Work out the finished part from the listing and answer in its coordinate system (mm). A direction names the side the tool comes from. Give positions to 0.01 mm unless a question says otherwise; leave off trailing zeros. Order: outer loops, then holes, each group sorted by start corner. A loop starts at its lowest first (then second) coordinate and runs counter-clockwise, first axis right, second up.
Autodesk Inventor part; units mm, degrees
ref_plane "YZ Plane" through (0, 0, 0) normal (1, 0, 0) x (0, 1, 0)
ref_plane "XZ Plane" through (0, 0, 0) normal (0, 1, 0) x (-1, 0, 0)
ref_plane "XY Plane" through (0, 0, 0) normal (0, 0, 1) x (1, 0, 0)
sketch "Sketch1" plane through (0, 0, 0) normal (0, 0, 1) x (1, 0, 0)
  circle A0 centre (-10, 0) radius 1.5
  circle A1 centre (10, 0) radius 1.5
  circle A2 centre (-10, -20) radius 1.5
  circle A3 centre (10, -20) radius 1.5
  line L0 (-15, 10) -> (15, 10)
  line L1 (15, 10) -> (15, -30)
  line L2 (15, -30) -> (-15, -30)
  line L3 (-15, -30) -> (-15, 10)
  point P0 (0, 0)
  dimension "d0" = 3
  dimension "d1" = 3
  dimension "d2" = 20
  dimension "d3" = 10
  dimension "d4" = 3
  dimension "d5" = 3
  dimension "d6" = 20
  dimension "d7" = 20
  dimension "d8" = 20
  dimension "d9" = 10
  dimension "d10" = 30
  dimension "d11" = 15
  dimension "d12" = 40
  dimension "d13" = 10
extrude "Extrusion1" add sketch "Sketch1" along normal blind 4
sketch "Sketch2" plane through (0, 0, 4) normal (0, 0, 1) x (1, 0, 0)
  line L0 (0, 15.4421) -> (0, -37.5419) construction
  line L1 (-4, 15.4421) -> (-4, -37.5419) construction
  line L2 (-15, -30) -> (15, -30) construction
  line L3 (15, 10) -> (-15, 10)
  line L4 (9, -30) -> (9, 10)
  line L5 (7, 10) -> (7, -30)
  line L6 (7, 10) -> (9, 10)
  line L7 (7, -30) -> (9, -30)
  line L8 (6.3, 15.4421) -> (6.3, 10) construction
  line L9 (6.3, -30) -> (6.3, -37.5419) construction
  line L10 (-15, 10) -> (-15, -30)
  point P0 (0, 0)
  dimension "d16" = 4
  dimension "d96" = 0
  dimension "d97" = 0
  dimension "d141" = 22
extrude "Extrusion2" add sketch "Sketch2" along normal blind 6
sketch "Sketch4" plane through (0, 0, 10) normal (0, 0, 1) x (1, 0, 0)
  circle A0 centre (10, 0) radius 2.75
  circle A1 centre (10, -20) radius 1.5
  circle A2 centre (10, -20) radius 2.75
  point P0 (0, 0)
  point P1 (8.5, 0)
  point P2 (8.5, -20)
  dimension "d37" = 5.5
  dimension "d38" = 5.5
extrude "Extrusion3" cut sketch "Sketch4" against normal up to surface (6 mm away) contours A0 | A1 | A2
sketch "Sketch5" plane through (0, 0, 4) normal (0, 0, 1) x (1, 0, 0)
  line L0 (-4, 15.4421) -> (-4, -37.5419) construction
  line L1 (15, -30) -> (-15, -30)
  line L2 (15, 10) -> (-15, 10)
  line L3 (-3.3, 10) -> (5, 10)
  line L4 (5, -30) -> (-3.3, -30)
  line L5 (-3.3, -30) -> (-3.3, 10)
  line L6 (-2, 7) -> (5, 7)
  line L7 (5, -27) -> (-2, -27)
  line L8 (-2, -27) -> (-2, 7)
  line L9 (5, 10) -> (5, 7)
  line L10 (5, -27) -> (5, -30)
  line L11 (7, 10) -> (7, -30)
  point P0 (0, 0)
  point P1 (6.3, 10)
  point P2 (6.3, -30)
  dimension "d111" = 0.7
  dimension "d112" = 3
  dimension "d115" = 3
  dimension "d116" = 1.3
  dimension "d117" = 2
  dimension "d118" = 2
  dimension "d139" = 0
  dimension "d140" = 0
extrude "Extrusion4" add sketch "Sketch5" along normal up to surface (6 mm away) contours L1 L5 L2 L9 L6 L8 L7 L10
sketch "Sketch8" plane through (0, 0, 0) normal (0, 0, -1) x (-1, 0, 0)
  line L0 (27, -15) -> (-27, -15)
  line L1 (-27, -15) -> (-27, -5)
  line L2 (-27, -5) -> (27, -5)
  line L3 (27, -5) -> (27, -15)
  line L4 (15, 10) -> (-15, 10)
  line L5 (-15, -30) -> (15, -30)
  circle A0 centre (23, -10) radius 1.5
  circle A1 centre (-23, -10) radius 1.5
  point P0 (0, 0)
  dimension "d77" = 10
  dimension "d78" = 40
  dimension "d79" = 15
  dimension "d80" = 3
  dimension "d81" = 3
  dimension "d82" = 46
  dimension "d83" = 54
  dimension "d84" = 23
  dimension "d85" = 27
extrude "Extrusion5" add sketch "Sketch8" against normal up to surface (4 mm away)
sketch "Sketch3" plane through (0, 0, 4) normal (0, 0, 1) x (1, 0, 0)
  circle A0 centre (2, -2) radius 1.25
  circle A1 centre (2, -15) radius 1.25
  line L0 (-15, -30) -> (15, -30)
  line L1 (15, 10) -> (-15, 10)
  point P0 (0, 0)
  point P1 (7, -30)
  point P2 (6.3, 10)
  dimension "d23" = 2.5
  dimension "d24" = 2.5
  dimension "d25" = 15
  dimension "d26" = 2
  dimension "d27" = 2
  dimension "d28" = 12
hole "Hole1" at (2, -2, 4) at (2, -15, 4) direction (0, 0, -1) diameter 2.5 end through all
fillet "Fillet5" [suppressed]
fillet "Fillet7" [suppressed]
sketch "Sketch11" plane through (0, 0, 0) normal (0, 0, -1) x (-1, 0, 0)
  line L0 (15, -15) -> (13.5, -15)
  line L1 (13.5, -5) -> (15, -5)
  line L2 (-15, -5) -> (-13.5, -5)
  line L3 (-13.5, -15) -> (-15, -15)
  line L4 (15, -30) -> (15, -15)
  line L5 (-15, -15) -> (-15, -30)
  line L6 (-15, 10) -> (-15, -5)
  line L7 (15, -5) -> (15, 10)
  line L8 (-15, -30) -> (-13.5, -30)
  line L9 (13.5, -30) -> (15, -30)
  line L10 (-13.5, -30) -> (-13.5, -15)
  line L11 (-13.5, -5) -> (-13.5, 10)
  line L12 (13.5, 10) -> (13.5, -5)
  line L13 (13.5, -15) -> (13.5, -30)
  line L14 (15, 10) -> (13.5, 10)
  line L15 (-15, 10) -> (15, 10)
  line L16 (-15, 10) -> (-13.5, 10)
  point P0 (0, 0)
  dimension "d121" = 27
extrude "Extrusion7" cut sketch "Sketch11" against normal through all
fillet "Fillet9" radius 3 12 edges at (-27, -15, 2) (-13.5, -30, 2) (13.5, -30, 2) (-27, -5, 2) (-13.5, -5, 2) (-13.5, 10, 2) (13.5, -15, 2) (27, -15, 2) (27, -5, 2) (13.5, -5, 2) (13.5, 10, 2) (-13.5, -15, 2)
sketch "Sketch12" plane through (4, -30, 4) normal (0, -1, 0) x (1, 0, 0)
  line L0 (1, 6) -> (-7.3, 6)
  circle A0 centre (-2, 3) radius 1.5
  line L1 (5, 0) -> (6.5, 0)
  line L2 (6.5, -4) -> (-14.5, -4)
  line L3 (6.5, 0) -> (6.5, -4)
  line L4 (-14.5, -4) -> (-14.5, 0)
  line L5 (-7.3, 0) -> (-7.3, 6)
  line L6 (-14.5, 0) -> (-7.3, 0)
  line L7 (5, 0) -> (5, 6)
  line L8 (3, 6) -> (5, 6)
  line L9 (3, 0) -> (3, 6)
  line L10 (1, 0) -> (3, 0)
  line L11 (1, 0) -> (1, 6)
  point P0 (-4, -4)
  dimension "d126" = 3
  dimension "d129" = 3
extrude "Extrusion8" [suppressed]
sketch "Sketch14" plane through (0, 0, 0) normal (0, 0, -1) x (-1, 0, 0)
  line L0 (10.5, 10) -> (-10.5, 10)
  line L1 (-1.2, 10) -> (1.2, 10)
  line L2 (1.2, 10) -> (1.2, 24)
  line L3 (1.2, 24) -> (-1.2, 24)
  line L4 (-1.2, 24) -> (-1.2, 10)
  point P0 (0, 0)
  dimension "d142" = 14
  dimension "d143" = 1.2
  dimension "d144" = 1.2
extrude "Extrusion10" add sketch "Sketch14" against normal blind 10
fillet "Fillet10" radius 3 2 edges at (-1.2, 10, 5) (1.2, 10, 5)
fillet "Fillet11" radius 1 2 edges at (-1.2, 24, 5) (1.2, 24, 5)
sketch "Sketch13" plane through (-10.5, -30, 0) normal (0, -1, 0) x (1, 0, 0)
  line L0 (21, 4) -> (21, 0)
  line L1 (0, 4) -> (21, 4)
  line L2 (0, 0) -> (0, 4)
  line L3 (21, 0) -> (0, 0)
  circle A0 centre (10.5, 2) radius 1.5
  point P0 (10.5, 0)
  dimension "d132" = 3
  dimension "d133" = 21
  dimension "d134" = 4
  dimension "d135" = 2
  dimension "d136" = 10.5
sketch "Sketch9" plane through (0, 0, 4) normal (0, 0, 1) x (1, 0, 0)
  circle A0 centre (-10, 0) radius 1.5
  circle A1 centre (2, -2) radius 1.25
  circle A2 centre (10, 0) radius 1.5
  circle A3 centre (23, -10) radius 1.5
  circle A4 centre (10, -20) radius 1.5
  circle A5 centre (2, -15) radius 1.25
  circle A6 centre (-10, -20) radius 1.5
  circle A7 centre (-23, -10) radius 1.5
  point P0 (0, 0)
equation "\"d7\" = d6"
equation "\"d8\" = d2"
equation "\"d37\" = d38"
equation "\"d115\" = d112"
equation "\"d79\" = -0.5 * d77 + 0.5 * d78"
properties part number "vertical carriage"
1. The part is cut by section D-D (y = 5). Write down the section's boundary in (x, z).
Findings below:
outline: (-13.5, 0) - (13.5, 0) - (13.5, 4) - (9, 4) - (9, 10) - (7, 10) - (7, 4) - (-2, 4) - (-2, 10) - (-3.3, 10) - (-3.3, 4) - (-13.5, 4) - close
2. The part is cut by section A-A (z = 5.75). Write down the section's boundary in (x, y).
Findings below:
outline: (-3.3, -30) - (5, -30) - (5, -27) - (-2, -27) - (-2, 7) - (5, 7) - (5, 10) - (4.2, 10) arc R3 cw to (1.2, 13) - (1.2, 23) arc R1 ccw to (0.2, 24) - (-0.2, 24) arc R1 ccw to (-1.2, 23) - (-1.2, 13) arc R3 cw to (-3.3, 10.14) - close; (7, -30) - (9, -30) - (9, -22.56) arc R2.75 cw to (9, -17.44) - (9, -2.56) arc R2.75 cw to (9, 2.56) - (9, 10) - (7, 10) - close
3. The part is cut by section B-B (y = -20). Write down the section's boundary in (x, z).
Findings below:
outline: (-13.5, 0) - (-11.5, 0) - (-11.5, 4) - (-13.5, 4) - close; (-8.5, 0) - (8.5, 0) - (8.5, 4) - (7.25, 4) - (7.25, 10) - (7, 10) - (7, 4) - (-2, 4) - (-2, 10) - (-3.3, 10) - (-3.3, 4) - (-8.5, 4) - close; (11.5, 0) - (13.5, 0) - (13.5, 4) - (11.5, 4) - close
4. Straight lines are drawn through the part: probe 1 along Y at (x, z) = (10, 1.05); probe 2 along Y at (x, z) = (-23, 1.5); probe 3 along X at (y, z) = (-9, 4.25). For each, find the intervals that lie inside material, in ascending order.
Findings below:
probe 1: y = -30 to -21.5, -18.5 to -1.5, 1.5 to 10
probe 2: y = -15 to -11.5, -8.5 to -5
probe 3: x = -3.3 to -2, 7 to 9
5. Which of the six approach directions +Z, -Z, +X, -X, +Y, -Y give full straight-line access (tool end or side, diameter ignored) to faces 1 (the face through (-13.5, 3, 2)), 2 (the face through (20, -15, 2)), 3 (the face through (1, 7, 7)), 4 (the face through (13.5, 2, 2))?
Findings below:
face 1: +Z, -Z, -X, +Y
face 2: +Z, -Z, +X, -Y
face 3: +Z
face 4: +Z, -Z, +X, +Y
6. The mould has two halves that part along X. Classify faces 5 (the face through (9, -10, 7)), 6 (the face through (2, -10, 4)), 7 (the face through (7.3, 10, 3.8)): pulls with the +X half, pulls with the -X half, needs draft (parallel to the pull), parting line crosses it, or undercut.
Findings below:
face 5: pulls with the +X half
face 6: undercut
face 7: needs draft
7. Given P1, Ø4, axis at x = 7, y = 12.5, coming from the -Z side; P2, Ø10, axis at x = 21.5, y = -0.5, coming from the +Z side; P3, Ø6, axis at y = -21.5, z = 9, coming from the +X side; P4, Ø3, axis at x = -21, z = 2.5, coming from the -Y side, each flat-ended and moving along its own axis, determine where each tip first touches the part or whether it passes through.
Findings below:
P1: passes through
P2: stops at z = 4
P3: stops at x = 9
P4: stops at y = -15
8. The part is cut by section C-C (x = -23). Write down the section's boundary in (y, z).
Findings below:
outline: (-15, 0) - (-11.5, 0) - (-11.5, 4) - (-15, 4) - close; (-8.5, 0) - (-5, 0) - (-5, 4) - (-8.5, 4) - close
